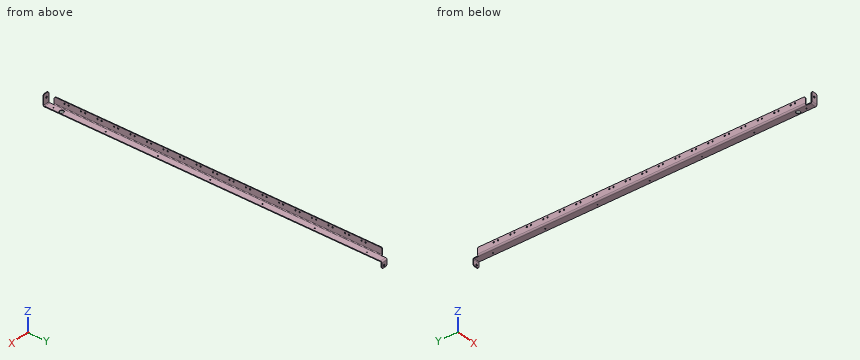
```python
from build123d import *

# Parameters (mm, degrees)
BASE_FLANGE1_DEPTH           = 1565.275
SKETCH6_W                    = 6.35
SKETCH6_H                    = 25.4
CUT_EXTRUDE1_DEPTH           = 50.8
EDGE_FLANGE1_STRIP_W         = 19.05
EDGE_FLANGE1_STRIP_H         = 3.175
EDGE_FLANGE1_STRIP_CUT_DEPTH = 28.575
EDGE_FLANGE1_DEPTH           = 28.575
FILLET1_R                    = 6.35
SKETCH10_R                   = 2.4511
SKETCH10_R_2                 = 9.525
CUT_EXTRUDE2_DEPTH           = 50.8
SKETCH11_R                   = 4.3688
CUT_EXTRUDE3_DEPTH           = 50.8
SKETCH12_R                   = 3.175
CUT_EXTRUDE4_DEPTH           = 50.8
EDGE_FLANGE3_STRIP_W         = 19.05
EDGE_FLANGE3_STRIP_H         = 3.175
EDGE_FLANGE3_STRIP_CUT_DEPTH = 28.575
EDGE_FLANGE3_DEPTH           = 28.575
FILLET2_R                    = 6.35
SKETCH21_R                   = 4.3688
CUT_EXTRUDE5_DEPTH           = 6.35


# Sheet-metal steps are written as plain solids
with BuildPart() as part:
    # Sketch1 → Base-Flange1 (new body)
    with BuildSketch(Plane(origin=(0, 0, 0), x_dir=(1, 0, 0), z_dir=(0, 1, 0))):
        with BuildLine():
            Line((0, -34.925), (0, -6.35))
            ThreePointArc((0, -6.35), (1.859871939, -1.859871939), (6.35, 0))
            Line((6.35, 0), (34.925, 0))
            Line((34.925, 0), (34.925, -3.175))
            Line((34.925, -3.175), (6.35, -3.175))
            ThreePointArc((6.35, -3.175), (4.10493597, -4.10493597), (3.175, -6.35))
            Line((3.175, -6.35), (3.175, -34.925))
            Line((3.175, -34.925), (0, -34.925))
        make_face()
    extrude(amount=BASE_FLANGE1_DEPTH)

    # Sketch6 → Cut-Extrude1 (cut)
    with BuildSketch(Plane(origin=(0, 0, 0), x_dir=(-1, 0, 0), z_dir=(0, 0, -1))):
        with Locations((-3.175, 12.7)):
            Rectangle(SKETCH6_W, SKETCH6_H)
        with Locations((-3.175, 1552.575)):
            Rectangle(SKETCH6_W, SKETCH6_H)
    extrude(amount=-CUT_EXTRUDE1_DEPTH, mode=Mode.SUBTRACT)

    # Edge-Flange1 strip (across the edge) → Edge-Flange1 strip cut (cut)
    with BuildSketch(Plane(origin=(6.35, 0, 3.175), x_dir=(0, 1, 0), z_dir=(1, 0, 0))):
        with Locations((-3.175, -1.5875)):
            Rectangle(EDGE_FLANGE1_STRIP_W, EDGE_FLANGE1_STRIP_H)
    extrude(amount=EDGE_FLANGE1_STRIP_CUT_DEPTH, mode=Mode.SUBTRACT)

    # Edge-Flange1 section (across the edge) → Edge-Flange1 (add)
    with BuildSketch(Plane(origin=(6.35, 0, 3.175), x_dir=(0, 1, 0), z_dir=(1, 0, 0))):
        with BuildLine():
            Line((0, 3.175), (0, 47.625))
            Line((0, 47.625), (3.175, 47.625))
            Line((3.175, 47.625), (3.175, 3.175))
            ThreePointArc((3.175, 3.175), (4.10493597, 0.92993597), (6.35, 0))
            Line((6.35, 0), (6.35, -3.175))
            ThreePointArc((6.35, -3.175), (1.859871939, -1.315128061), (0, 3.175))
        make_face()
    extrude(amount=EDGE_FLANGE1_DEPTH)

    # Fillet1
    fillet1_edges = [part.edges().sort_by_distance(p)[0] for p in [
        (6.35, 1.5875, 50.8),
        (34.925, 1.5875, 50.8),
        (1.5875, 25.4, 34.925),
        (1.5875, 1539.875, 34.925),
    ]]
    fillet(fillet1_edges, radius=FILLET1_R)

    # Sketch10 → Cut-Extrude2 (cut)
    with BuildSketch(Plane.XY.offset(3.175)):
        with Locations((22.225, 38.1)):
            Circle(SKETCH10_R)
        with Locations((22.225, 279.4)):
            Circle(SKETCH10_R)
        with Locations((22.225, 520.7)):
            Circle(SKETCH10_R)
        with Locations((22.225, 762)):
            Circle(SKETCH10_R)
        with Locations((22.225, 1003.3)):
            Circle(SKETCH10_R)
        with Locations((22.225, 1244.6)):
            Circle(SKETCH10_R)
        with Locations((22.225, 1485.9)):
            Circle(SKETCH10_R)
        with Locations((22.225, 76.2)):
            Circle(SKETCH10_R_2)
    extrude(amount=-CUT_EXTRUDE2_DEPTH, mode=Mode.SUBTRACT)

    # Sketch11 → Cut-Extrude3 (cut)
    with BuildSketch(Plane.XZ):
        with Locations(Location((19.05, 31.75, 0), (0, 0, 270))):
            Circle(SKETCH11_R)
    extrude(amount=-CUT_EXTRUDE3_DEPTH, mode=Mode.SUBTRACT)

    # Sketch12 → Cut-Extrude4 (cut)
    with BuildSketch(Plane(origin=(3.175, 0, 0), x_dir=(0, 0, -1), z_dir=(1, 0, 0))):
        with Locations((-25.4, 73.025)):
            Circle(SKETCH12_R)
        with Locations((-25.4, 92.075)):
            Circle(SKETCH12_R)
        with Locations((-25.4, 149.225)):
            Circle(SKETCH12_R)
        with Locations((-25.4, 168.275)):
            Circle(SKETCH12_R)
        with Locations((-25.4, 225.425)):
            Circle(SKETCH12_R)
        with Locations((-25.4, 244.475)):
            Circle(SKETCH12_R)
        with Locations((-25.4, 301.625)):
            Circle(SKETCH12_R)
        with Locations((-25.4, 320.675)):
            Circle(SKETCH12_R)
        with Locations((-25.4, 377.825)):
            Circle(SKETCH12_R)
        with Locations((-25.4, 396.875)):
            Circle(SKETCH12_R)
        with Locations((-25.4, 454.025)):
            Circle(SKETCH12_R)
        with Locations((-25.4, 473.075)):
            Circle(SKETCH12_R)
        with Locations((-25.4, 530.225)):
            Circle(SKETCH12_R)
        with Locations((-25.4, 549.275)):
            Circle(SKETCH12_R)
        with Locations((-25.4, 606.425)):
            Circle(SKETCH12_R)
        with Locations((-25.4, 625.475)):
            Circle(SKETCH12_R)
        with Locations((-25.4, 682.625)):
            Circle(SKETCH12_R)
        with Locations((-25.4, 701.675)):
            Circle(SKETCH12_R)
        with Locations((-25.4, 758.825)):
            Circle(SKETCH12_R)
        with Locations((-25.4, 777.875)):
            Circle(SKETCH12_R)
        with Locations((-25.4, 835.025)):
            Circle(SKETCH12_R)
        with Locations((-25.4, 854.075)):
            Circle(SKETCH12_R)
        with Locations((-25.4, 911.225)):
            Circle(SKETCH12_R)
        with Locations((-25.4, 930.275)):
            Circle(SKETCH12_R)
        with Locations((-25.4, 987.425)):
            Circle(SKETCH12_R)
        with Locations((-25.4, 1006.475)):
            Circle(SKETCH12_R)
        with Locations((-25.4, 1063.625)):
            Circle(SKETCH12_R)
        with Locations((-25.4, 1082.675)):
            Circle(SKETCH12_R)
        with Locations((-25.4, 1139.825)):
            Circle(SKETCH12_R)
        with Locations((-25.4, 1158.875)):
            Circle(SKETCH12_R)
        with Locations((-25.4, 1216.025)):
            Circle(SKETCH12_R)
        with Locations((-25.4, 1235.075)):
            Circle(SKETCH12_R)
        with Locations((-25.4, 1292.225)):
            Circle(SKETCH12_R)
        with Locations((-25.4, 1311.275)):
            Circle(SKETCH12_R)
        with Locations((-25.4, 1368.425)):
            Circle(SKETCH12_R)
        with Locations((-25.4, 1387.475)):
            Circle(SKETCH12_R)
        with Locations((-25.4, 1444.625)):
            Circle(SKETCH12_R)
        with Locations((-25.4, 1463.675)):
            Circle(SKETCH12_R)
    extrude(amount=-CUT_EXTRUDE4_DEPTH, mode=Mode.SUBTRACT)

    # Edge-Flange3 strip (across the edge) → Edge-Flange3 strip cut (cut)
    with BuildSketch(Plane(origin=(6.35, 1565.275, 0), x_dir=(0, -1, 0), z_dir=(1, 0, 0))):
        with Locations((-3.175, -1.5875)):
            Rectangle(EDGE_FLANGE3_STRIP_W, EDGE_FLANGE3_STRIP_H)
    extrude(amount=EDGE_FLANGE3_STRIP_CUT_DEPTH, mode=Mode.SUBTRACT)

    # Edge-Flange3 section (across the edge) → Edge-Flange3 (add)
    with BuildSketch(Plane(origin=(6.35, 1565.275, 0), x_dir=(0, -1, 0), z_dir=(1, 0, 0))):
        with BuildLine():
            Line((0, 3.175), (0, 28.575))
            Line((0, 28.575), (3.175, 28.575))
            Line((3.175, 28.575), (3.175, 3.175))
            ThreePointArc((3.175, 3.175), (4.10493597, 0.92993597), (6.35, 0))
            Line((6.35, 0), (6.35, -3.175))
            ThreePointArc((6.35, -3.175), (1.859871939, -1.315128061), (0, 3.175))
        make_face()
    extrude(amount=EDGE_FLANGE3_DEPTH)

    # Fillet2
    fillet2_edges = [part.edges().sort_by_distance(p)[0] for p in [
        (6.35, 1563.6875, -28.575),
        (34.925, 1563.6875, -28.575),
    ]]
    fillet(fillet2_edges, radius=FILLET2_R)

    # Sketch21 → Cut-Extrude5 (cut)
    with BuildSketch(Plane(origin=(0, 1565.275, 0), x_dir=(1, 0, 0), z_dir=(0, 1, 0))):
        with Locations(Location((22.225, 19.05, 0), (0, 0, 270))):
            Circle(SKETCH21_R)
    extrude(amount=-CUT_EXTRUDE5_DEPTH, mode=Mode.SUBTRACT)


solid = part.part
```
The listing builds one solid part. Answer for the finished solid, in the listing's coordinates (mm). Round coordinates to 2 decimals unless told otherwise and drop trailing zeros. Write each loop counter-clockwise with the first axis right and the second up, starting at its lowest first coordinate (ties: lowest second). Pieces come first, ordered by that corner, then holes. Notation, with made-up numbers: (-12, 84) -> (2, 84) arc R17 ccw to (2, 102) -> close; hole circle Ø11 at (31.5, -21). An arc over 180 degrees is marked (long way). Answer as a JSON object with one key per item and string values. Group by question number.
Q1. Section A-A (y = 436) is taken. Write down the section's boundary in (x, z) (3 decimals).
Q2. Straight lines are drawn through the part: line 1 along X through (y, z) = (1564, -19) (3 decimals); line 2 along X through (y, z) = (370, 5); line 3 along Y through (x, z) = (31, 27) (3 decimals). For each, find the intervals that lie inside material, in ascending order.
Q3. Each of these flat-tipped pins is pushed along its axis until it touches: pin 1 Ø6 at (x, y) = (9.5, 734) entering from +Z (3 decimals); pin 2 Ø2 at (x, y) = (27.5, 1287) entering from -Z; pin 3 Ø10 at (y, z) = (1235.075, 25.4) entering from +X (3 decimals). Where does it stop, or does it pass through?
Check values:
{
 "1": {"outline": "(0, 6.35) arc R6.35 ccw to (6.35, 0) -> (34.925, 0) -> (34.925, 3.175) -> (6.35, 3.175) arc R3.175 cw to (3.175, 6.35) -> (3.175, 34.925) -> (0, 34.925) -> close"},
 "2": {"line 1": "6.35 to 17.856, 26.594 to 34.925", "line 2": "0.15 to 3.48", "line 3": "0 to 3.175"},
 "3": {"pin 1": "z = 3.175", "pin 2": "z = 0", "pin 3": "x = 3.175"}
}
